from build123d import *

# Parameters (mm, degrees)
SKETCH1_W           = 98
SKETCH1_H           = 42
BOSS_EXTRUDE1_DEPTH = 20
SKETCH2_W           = 70
SKETCH2_H           = 9
CUT_EXTRUDE1_DEPTH  = 68.564783726
SKETCH3_W           = 42
SKETCH3_H           = 42
BOSS_EXTRUDE2_DEPTH = 7
FILLET1_RADIUS      = 21
FILLET1_LENGTH      = 14
SKETCH4_R           = 10
CUT_EXTRUDE2_DEPTH  = 87.145226217
SKETCH5_R           = 7.424250223
CUT_EXTRUDE5_DEPTH  = 68.867518004
FILLET2_R           = 5


with BuildPart() as part:
    # Sketch1 → Boss-Extrude1 (new body)
    with BuildSketch(Plane(origin=(0, 0, 0), x_dir=(1, 0, 0), z_dir=(0, 1, 0))):
        Rectangle(SKETCH1_W, SKETCH1_H)
    extrude(amount=BOSS_EXTRUDE1_DEPTH)

    # Sketch2 → Cut-Extrude1 (cut, through all)
    with BuildSketch(Plane.XY.offset(21)):
        with Locations((0, 4.5)):
            Rectangle(SKETCH2_W, SKETCH2_H)
    extrude(amount=-CUT_EXTRUDE1_DEPTH, mode=Mode.SUBTRACT)

    # Sketch3 → Boss-Extrude2 (add, symmetric)
    with BuildSketch(Plane(origin=(0, 0, 0), x_dir=(0, 0, -1), z_dir=(1, 0, 0))):
        with Locations((0, 41)):
            Rectangle(SKETCH3_W, SKETCH3_H)
    extrude(amount=BOSS_EXTRUDE2_DEPTH, both=True)

    # Fillet1: full round fillet: the end face becomes a half cylinder, R = half its width
    fillet1_face = Plane((0, 62, 0), x_dir=(1, 0, 0), z_dir=(0, 1, 0))  # on the end face: x along it, z out of the body
    fillet1_slab = fillet1_face.offset(-FILLET1_RADIUS / 2) * Box(FILLET1_LENGTH, 2 * FILLET1_RADIUS, FILLET1_RADIUS, mode=Mode.PRIVATE)  # the body's end, R deep
    fillet1_round = Plane((0, 41, 0), x_dir=(0, 1, 0), z_dir=(1, 0, 0)) * Cylinder(FILLET1_RADIUS, FILLET1_LENGTH, mode=Mode.PRIVATE)  # its axis R under the face
    add(fillet1_slab - fillet1_round, mode=Mode.SUBTRACT)

    # Sketch4 → Cut-Extrude2 (cut, through all)
    with BuildSketch(Plane(origin=(7, 0, 0), x_dir=(0, 0, -1), z_dir=(1, 0, 0))):
        with Locations((0, 41)):
            Circle(SKETCH4_R)
    extrude(amount=-CUT_EXTRUDE2_DEPTH, mode=Mode.SUBTRACT)

    # Sketch5 → Cut-Extrude5 (cut, through all)
    with BuildSketch(Plane(origin=(0, 20, 0), x_dir=(1, 0, 0), z_dir=(0, 1, 0))):
        with Locations(Location((-25, 0, 0), (0, 0, 270))):
            Circle(SKETCH5_R)
        with Locations(Location((25, 0, 0), (0, 0, 270))):
            Circle(SKETCH5_R)
    extrude(amount=-CUT_EXTRUDE5_DEPTH, mode=Mode.SUBTRACT)

    # Fillet2
    fillet2_edges = [part.edges().sort_by_distance(p)[0] for p in [
        (-49, 20, 0),
        (-7, 20, 0),
        (7, 20, 0),
        (49, 20, 0),
    ]]
    fillet(fillet2_edges, radius=FILLET2_R)


solid = part.part
Read the model definition and answer for the solid it produces. Units are mm, in the model's axes. A direction names the side the tool comes from. Round coordinates to 2 decimals unless told otherwise and drop trailing zeros. Write each loop counter-clockwise with the first axis right and the second up, starting at its lowest first coordinate (ties: lowest second). Pieces come first, ordered by that corner, then holes. Notation, with made-up numbers: M -31,-24.5 L 17,-24.5 A21 cw 17,5.5 Z; hole C 64.25,88 d3. An arc over 180 degrees is marked long. Use a Markdown table: item, result.
1) The part is cut by section A-A (x = -25). Write down the section's boundary in (y, z).
Answers follow:
| item | result |
|---|---|
| outline | M 9,-21 L 20,-21 L 20,-7.42 L 9,-7.42 Z; M 9,7.42 L 20,7.42 L 20,21 L 9,21 Z |
2) Flat-ended cylindrical pins translate along their axes: pin 1 (1.5 mm diameter, centred on y = 32, z = 16, fed in from +X); pin 2 (16 mm diameter, centred on x = -32.5, z = -7, fed in from +Y); pin 3 (24 mm diameter, centred on x = 25, z = 0, fed in from -Y); pin 4 (4 mm diameter, centred on y = 22.5, z = 6, fed in from +X). Find the tip coordinate at first contact, or state that the pin passes through.
Answers follow:
| item | result |
|---|---|
| pin 1 | stops at x = 7 |
| pin 2 | stops at y = 20 |
| pin 3 | stops at y = 0 |
| pin 4 | stops at x = 9.82 |
3) The part is cut by section B-B (z = 0). Write down the section's boundary in (x, y).
Answers follow:
| item | result |
|---|---|
| outline | M -49,0 L -35,0 L -35,9 L -32.42,9 L -32.42,20 L -44,20 A5 ccw -49,15 Z; M -17.58,9 L 17.58,9 L 17.58,20 L 12,20 A5 cw 7,25 L 7,31 L -7,31 L -7,25 A5 cw -12,20 L -17.58,20 Z; M -7,51 L 7,51 L 7,62 L -7,62 Z; M 32.42,9 L 35,9 L 35,0 L 49,0 L 49,15 A5 ccw 44,20 L 32.42,20 Z |
4) A tool of negligible diameter and unlimited length cuts with its end or side. For faces 1 (the flat face through (-35, 4, 0)), 2 (the flat face through (0, 13, 21)), 3 (the flat face through (7, 44, 10)), 4 (the flat face through (-7, 44, 10)), 5 (the flat face through (0, 13, -21)), from which of +Z, -Z, +X, -X, +Y, -Y can it reach the whole face along a straight path? Write none if from no direction.
Answers follow:
| item | result |
|---|---|
| face 1 | +Z, -Z, -Y |
| face 2 | +Z, +X, -X, +Y, -Y |
| face 3 | +Z, -Z, +X, +Y |
| face 4 | +Z, -Z, -X, +Y |
| face 5 | -Z, +X, -X, +Y, -Y |
5) The part is cut by section D-D (x = 39). Write down the section's boundary in (y, z), plus the area to 3 significant figures.
Answers follow:
| item | result |
|---|---|
| outline | M 0,-21 L 20,-21 L 20,21 L 0,21 Z |
| area | 840 mm2 |
6) The part is cut by section C-C (y = 38). Write down the section's boundary in (x, z).
Answers follow:
| item | result |
|---|---|
| outline | M -7,-21 L 7,-21 L 7,-9.54 L -7,-9.54 Z; M -7,9.54 L 7,9.54 L 7,21 L -7,21 Z |
7) Straight lines are drawn through the part: line 1 along X through (y, z) = (13, 0); line 2 along Y through (x, z) = (0, 0); line 3 along X through (y, z) = (32.5, 13). For each, find the intervals that lie inside material, in ascending order. Write a range as [from, to].
Answers follow:
| item | result |
|---|---|
| line 1 | x = [-49, -32.42], [-17.58, 17.58], [32.42, 49] |
| line 2 | y = [9, 31], [51, 62] |
| line 3 | x = [-7, 7] |
8) For a pull along Y with two mould halves and no side action, classify faces 6 (the flat face through (0, 9, 0)), 7 (the cylindrical face through (-48, 18, 0)), 8 (the cylindrical face through (0.1, 31.24, 2.17)), 9 (the flat face through (35, 4, 0)) as pulls with the +Y half, pulls with the -Y half, needs draft (parallel to the pull), parting line crosses it, or undercut.
Answers follow:
| item | result |
|---|---|
| face 6 | pulls with the -Y half |
| face 7 | pulls with the +Y half |
| face 8 | undercut |
| face 9 | needs draft |
